Design review of the part built by this model. Coordinates are the model's own, in mm. A direction names the side the tool comes from. Give positions to 0.01 mm unless a question says otherwise; leave off trailing zeros. Write each loop counter-clockwise with the first axis right and the second up, starting at its lowest first coordinate (ties: lowest second). Pieces come first, ordered by that corner, then holes. Notation, with made-up numbers: M 17.5,33.5 L 28.5,33.5 A13 ccw 28.5,57.5 Z; hole C 22,-32 d3. An arc over 180 degrees is marked long. Answer in a Markdown table with one row per item.
```python
from build123d import *

# Parameters (mm, degrees)
ESQUISSE1_W        = 61.6
ESQUISSE1_H        = 26.2
BOSS_EXTRU_1_DEPTH = 1.6
D_GAGEMENT_M31_D   = 3.4
ESQUISSE5_R        = 3.691889044
ESQUISSE5_W        = 7.8
ESQUISSE5_H        = 9.9
ESQUISSE5_W_2      = 9.402735495
ESQUISSE5_H_2      = 4.28999807
ESQUISSE5_W_3      = 5.40657291
ESQUISSE5_H_3      = 11.812186467
BOSS_EXTRU_2_DEPTH = 10.5


with BuildPart() as part:
    # Esquisse1 → Boss.-Extru.1 (new body)
    with BuildSketch(Plane.XY):
        Rectangle(ESQUISSE1_W, ESQUISSE1_H)
    extrude(amount=BOSS_EXTRU_1_DEPTH)

    # Dégagement M31 (through all)
    with Locations(Plane.XY.offset(1.6)):
        with Locations((-28.25, 10.5), (28.25, 10.5), (28.25, -10.5), (-28.25, -10.5)):
            Hole(D_GAGEMENT_M31_D / 2)

    # Esquisse5 → Boss.-Extru.2 (add)
    with BuildSketch(Plane.XY.offset(1.6)):
        with Locations(Location((-15.725040559, -6.949067891, 0), (0, 0, 180))):
            Circle(ESQUISSE5_R)
        with Locations(Location((15.725040559, -6.949067891, 0), (0, 0, 180))):
            Circle(ESQUISSE5_R)
        with Locations((-26.443929164, 0)):
            Rectangle(ESQUISSE5_W, ESQUISSE5_H)
        with Locations((26.443929164, 0)):
            Rectangle(ESQUISSE5_W, ESQUISSE5_H)
        with Locations((6.557373451, 8.653596323)):
            Rectangle(ESQUISSE5_W_2, ESQUISSE5_H_2)
        with Locations((4.843443338, -4.157630791)):
            Rectangle(ESQUISSE5_W_3, ESQUISSE5_H_3)
        with Locations((-6.557373451, 8.653596323)):
            Rectangle(ESQUISSE5_W_2, ESQUISSE5_H_2)
    extrude(amount=BOSS_EXTRU_2_DEPTH)


solid = part.part
```
1) Add section B-B (z = 7.25). Write out the cut boundary in (x, y), and give its area (3 significant figures).
Geometry says:
| item | result |
|---|---|
| outline | M -30.34,-4.95 L -22.54,-4.95 L -22.54,4.95 L -30.34,4.95 Z; C -15.73,-6.95 d7.38; M -11.26,6.51 L -1.86,6.51 L -1.86,10.8 L -11.26,10.8 Z; M 1.86,6.51 L 11.26,6.51 L 11.26,10.8 L 1.86,10.8 Z; M 2.14,-10.06 L 7.55,-10.06 L 7.55,1.75 L 2.14,1.75 Z; C 15.73,-6.95 d7.38; M 22.54,-4.95 L 30.34,-4.95 L 30.34,4.95 L 22.54,4.95 Z |
| area | 385 mm^2 |
2) Add section A-A (x = -28.25). Write out the cut boundary in (y, z), and give its area (3 significant figures).
Geometry says:
| item | result |
|---|---|
| outline | M -13.1,0 L -12.2,0 L -12.2,1.6 L -13.1,1.6 Z; M -8.8,0 L 8.8,0 L 8.8,1.6 L 4.95,1.6 L 4.95,12.1 L -4.95,12.1 L -4.95,1.6 L -8.8,1.6 Z; M 12.2,0 L 13.1,0 L 13.1,1.6 L 12.2,1.6 Z |
| area | 135 mm^2 |
3) To check wall thickness, follow probe 1 along Y at (x, z) = (-28.25, 0.85); probe 2 along X at (y, z) = (-8.25, 7.25); probe 3 along X at (y, z) = (9, 3.5). State the ranges of each line that lie inside material, in increasing order. Write a range as [from, to].
Geometry says:
| item | result |
|---|---|
| probe 1 | [-13.1, -12.2], [-8.8, 8.8], [12.2, 13.1] |
| probe 2 | [-19.18, -12.27], [2.14, 7.55], [12.27, 19.18] |
| probe 3 | [-11.26, -1.86], [1.86, 11.26] |
4) For faces 1 (the face through (2.14, -4, 7)), 2 (the face through (-17.429, -3.674, 6.776)), 3 (the face through (1.856, 9, 7)), 4 (the face through (-7, 10.799, 7)), list the 3-axis set-ups (+Z, -Z, +X, -X, +Y, -Y) from which the entire face can be reached by the end or side of a thin tool; tool diameter is ignored.
Geometry says:
| item | result |
|---|---|
| face 1 | +Z, -Y |
| face 2 | +Z |
| face 3 | +Z, +Y, -Y |
| face 4 | +Z, +X, -X, +Y |
5) Insertion check: P1, Ø4.5, axis at x = 3.5, z = 6.5, coming from the -Y side; P2, Ø4.5, axis at y = 8.5, z = 6, coming from the -X side; P3, Ø5, axis at x = -3.5, z = 8.5, coming from the +Y side. Each pin has a flat end and moves straight along its axis. Give the tip position at first contact, or say it passes through.
Geometry says:
| item | result |
|---|---|
| P1 | y = -10.06 |
| P2 | x = -11.26 |
| P3 | y = 10.8 |
6) The part is to be moulded in two halves that separate along X. For faces 5 (the face through (26.7, -11.2, 0.8)), 6 (the face through (-26, 4.95, 7)), 7 (the face through (30.8, 0, 1)), say which applies: released by +X, released by -X, zero draft, split by the parting line, or undercut.
Geometry says:
| item | result |
|---|---|
| face 5 | undercut |
| face 6 | zero draft |
| face 7 | released by +X |
7) Add section C-C (x = -9). Write out the cut boundary in (y, z).
Geometry says:
| item | result |
|---|---|
| outline | M -13.1,0 L 13.1,0 L 13.1,1.6 L 10.8,1.6 L 10.8,12.1 L 6.51,12.1 L 6.51,1.6 L -13.1,1.6 Z |
8) Add section D-D (x = 4.5). Write out the cut boundary in (y, z).
Geometry says:
| item | result |
|---|---|
| outline | M -13.1,0 L 13.1,0 L 13.1,1.6 L 10.8,1.6 L 10.8,12.1 L 6.51,12.1 L 6.51,1.6 L 1.75,1.6 L 1.75,12.1 L -10.06,12.1 L -10.06,1.6 L -13.1,1.6 Z |
